Autodesk Inventor part; units mm, degrees
ref_plane "YZ Plane" through (0, 0, 0) normal (1, 0, 0) x (0, 1, 0)
ref_plane "XZ Plane" through (0, 0, 0) normal (0, 1, 0) x (-1, 0, 0)
ref_plane "XY Plane" through (0, 0, 0) normal (0, 0, 1) x (1, 0, 0)
sketch "スケッチ1" plane through (0, 0, 0) normal (1, 0, 0) x (0, 1, 0)
  circle A0 centre (0, 0) radius 9
  circle A1 centre (0, 0) radius 6.5
  dimension "d0" = 18
  dimension "d1" = 13
extrude "押し出し1" add sketch "スケッチ1" against normal blind 150
sketch "スケッチ2" plane through (0, 0, 0) normal (0, 0, 1) x (1, 0, 0)
  point P0 (0, 0)
sketch "スケッチ3" plane through (0, 0, 0) normal (0, 0, 1) x (1, 0, 0)
  line L0 (0, 0) -> (0, 6)
  line L1 (0, -9) -> (0, 9)
  line L2 (0, 0) -> (0, -6)
  line L3 (0, -6) -> (-6, -6)
  line L4 (-6, -6) -> (-6, 6)
  line L5 (-6, 6) -> (0, 6)
  dimension "d4" = 6
  dimension "d5" = 6
  dimension "d6" = 6
extrude "押し出し2" cut sketch "スケッチ3" along normal mid plane 150
sketch "スケッチ4" plane through (0, 0, 0) normal (0, 0, 1) x (1, 0, 0)
  line L0 (-6, -6) -> (-6, 6)
  circle A0 centre (-6, 0) radius 6
  point P0 (0, 0)
extrude "押し出し3" cut sketch "スケッチ4" along normal mid plane 150 contours A0 L0 picked at (-9.4508, 1.581)
sketch "スケッチ5" plane through (0, 0, 0) normal (0, 0, 1) x (1, 0, 0)
  circle A0 centre (-140, 0) radius 1.5
  point P0 (0, 0)
  dimension "d11" = 3
extrude "押し出し4" cut sketch "スケッチ5" along normal mid plane 150
thread "ねじ1"
thread "ねじ2"
properties part number "vp13_150" material "PVC 配管"
Check sheet for the modelled part. Datum: model origin and axes. Units: mm. A direction names the side the tool comes from. Give positions to 0.01 mm unless a question says otherwise; leave off trailing zeros. Order: outer loops, then holes, each group sorted by start corner. A loop starts at its lowest first (then second) coordinate and runs counter-clockwise, first axis right, second up. Notation, with made-up numbers: M 72.5,-38.75 L 87.5,-38.75 A15 ccw 87.5,-25.75 Z; hole C -29.5,-26 d7. An arc over 180 degrees is marked long. Answer in a Markdown table with one row per item.
1) Release check for a two-part mould opening along Y. For faces 3 (the cylindrical face through (-141.5, 0.07, -7.64)), 4 (the flat face through (-150, 3, -6)), 5 (the flat face through (-3, -6, 5)), 6 (the cylindrical face through (-73.95, -1.951, -8.786)) record: +Y half, -Y half, draft (parallel to the pull), parting line (faces both ways), or undercut.
Filled sheet:
| item | result |
|---|---|
| face 3 | undercut |
| face 4 | draft |
| face 5 | undercut |
| face 6 | parting line |
2) Cross-section at D-D, the plane x = -42. Enter the section's corners in (y, z).
Filled sheet:
| item | result |
|---|---|
| outline | C 0,0 d18; hole C 0,0 d13 |
3) Cross-section at B-B, the plane x = -140. Enter the section's corners in (y, z), plus the area to 3 significant figures.
Filled sheet:
| item | result |
|---|---|
| outline | M -1.5,-8.87 L -1.5,-6.32 A6.5 cw -1.5,6.32 L -1.5,8.87 A9 ccw Z; M 1.5,-8.87 A9 ccw 1.5,8.87 L 1.5,6.32 A6.5 cw 1.5,-6.32 Z |
| area | 107 mm2 |
4) Cross-section at A-A, the plane y = 0. Enter the section's corners in (x, z).
Filled sheet:
| item | result |
|---|---|
| outline | M -150,-9 L -141.5,-9 L -141.5,-6.5 L -150,-6.5 Z; M -150,6.5 L -141.5,6.5 L -141.5,9 L -150,9 Z; M -138.5,-9 L -12,-9 L -12,-6.5 L -138.5,-6.5 Z; M -138.5,6.5 L -12,6.5 L -12,9 L -138.5,9 Z |
5) Access from +Z, -Z, +X, -X, +Y, -Y to the whole of each face (thin tool, end or side, straight path). Record for faces 1 (the flat face through (-3, 6, -5)), 2 (the cylindrical face through (-73.95, 2.999, -5.767)).
Filled sheet:
| item | result |
|---|---|
| face 1 | +Z, -Z, +X |
| face 2 | +X, -X |
6) Gauge pin test, flat ends, axial feed: P1, Ø1, axis at x = -55.5, z = -1, coming from the -Y side; P2, Ø2, axis at x = -2, z = 5.5, coming from the +Y side; P3, Ø1.8, axis at x = -140, y = 0, coming from the -Z side; P4, Ø8, axis at y = -6.5, z = 3, coming from the +X side. Record the tip position at first contact, or that the pin passes through.
Filled sheet:
| item | result |
|---|---|
| P1 | stops at y = -8.99 |
| P2 | stops at y = 7.79 |
| P3 | passes through |
| P4 | stops at x = 0 |
7) Cross-section at C-C, the plane z = 0. Enter the section's corners in (x, y), plus the area to 3 significant figures.
Filled sheet:
| item | result |
|---|---|
| outline | M -150,-9 L 0,-9 L 0,-6.5 L -150,-6.5 Z; M -150,6.5 L 0,6.5 L 0,9 L -150,9 Z |
| area | 750 mm2 |
8) Thickness scan on L1, parallel to Y at x = -94, z = 0.5; L2, parallel to X at y = 0, z = -8.4. Record the ranges inside material, lowest first. Write a range as [from, to].
Filled sheet:
| item | result |
|---|---|
| L1 | y = [-8.99, -6.48], [6.48, 8.99] |
| L2 | x = [-150, -141.5], [-138.5, -12] |
